The listing builds one solid part. Answer for the finished solid, in the listing's coordinates (mm). A direction names the side the tool comes from. Give positions to 0.01 mm unless a question says otherwise; leave off trailing zeros. Order: outer loops, then holes, each group sorted by start corner. A loop starts at its lowest first (then second) coordinate and runs counter-clockwise, first axis right, second up. Notation, with made-up numbers: M 24.5,3 L 49.5,3 A27 cw 49.5,29 Z; hole C -30.5,47.5 d2. An arc over 180 degrees is marked long. Answer as a JSON object with one key per item and string values. Group by question number.
```python
from build123d import *

# Parameters (mm, degrees)
F0_R     = 13.3
F0_R_2   = 11.5
F1_DEPTH = 2.2
F2_R     = 13.3
F2_R_2   = 11.5
F2_R_3   = 9.5
F3_DEPTH = 1
F4_R     = 11.5
F4_R_2   = 10.9
F5_DEPTH = 1


with BuildPart() as f1:
    # F0 (on Top) → F1 (new body)
    with BuildSketch(Plane.XY):
        Circle(F0_R)
        Circle(F0_R_2, mode=Mode.SUBTRACT)
    extrude(amount=F1_DEPTH)

    # F2 (on face) → F3 (join)
    with BuildSketch(Plane.XY.offset(2.2)):
        Circle(F2_R)
        Circle(F2_R_2, mode=Mode.SUBTRACT)
        Circle(F2_R_2)
        Circle(F2_R_3, mode=Mode.SUBTRACT)
    extrude(amount=F3_DEPTH)

    # F4 (on face) → F5 (join)
    with BuildSketch(Plane(origin=(0, 0, 0), x_dir=(1, 0, 0), z_dir=(0, 0, -1))):
        Circle(F4_R)
        Circle(F4_R_2, mode=Mode.SUBTRACT)
    extrude(amount=-F5_DEPTH)


solid = f1.part
```
Item 1: A flat-ended cylindrical pin translates along its axis: P1, Ø10, axis at x = 0, y = -7.5, coming from the -Z side. Find the tip coordinate at first contact, or state that the pin passes through.
Item 2: Section C-C (z = 1.55) is taken. Determine the outline of the cut face in (x, y).
Item 3: Consider probe 1 along Y at (x, z) = (0, 0.3); probe 2 along Y at (x, z) = (0, 1.8); probe 3 along Z at (x, y) = (-8.5, -5.75). Determine where each line is inside the solid, lowest interval first. Write a range as from..to.
Item 4: Section A-A (y = 0) is taken. Determine the outline of the cut face in (x, z).
Item 5: A tool of negligible diameter and unlimited length cuts with its end or side. For faces 1 (the cylindrical face through (-1.5, 11.4, 1.6)), 2 (the flat face through (9, -6, 3.2)), from which of +Z, -Z, +X, -X, +Y, -Y can it reach the whole face along a straight path? Write none if from no direction.
Item 6: Determine the mould class of faces 3 (the cylindrical face through (10.4, -3.27, 0.49)), 4 (the cylindrical face through (6.14, -11.8, 1.58)), 5 (the flat face through (-2, -11, 0)) for opening direction Y: released by +Y, released by -Y, zero draft, split by the parting line, or undercut.
Values found:
{
 "1": {"P1": "stops at z = 0"},
 "2": {"outline": "C 0,0 d26.6; hole C 0,0 d23"},
 "3": {"probe 1": "y = -13.3..-10.9, 10.9..13.3", "probe 2": "y = -13.3..-11.5, 11.5..13.3", "probe 3": "z = 2.2..3.2"},
 "4": {"outline": "M -13.3,0 L -10.9,0 L -10.9,1 L -11.5,1 L -11.5,2.2 L -9.5,2.2 L -9.5,3.2 L -13.3,3.2 Z; M 9.5,2.2 L 11.5,2.2 L 11.5,1 L 10.9,1 L 10.9,0 L 13.3,0 L 13.3,3.2 L 9.5,3.2 Z"},
 "5": {"face 1": "none", "face 2": "+Z, +X, -X, +Y, -Y"},
 "6": {"face 3": "undercut", "face 4": "split by the parting line", "face 5": "zero draft"}
}
